from build123d import *

# Parameters (mm, degrees)
EXTRUDE_DEPTH                  = 30
EXTRUDE_ONTO_SKETCH_ROLL_ANGLE = 90


with BuildPart() as part:
    # Sketch as drawn → Extrude (new)
    with BuildSketch(Plane.XY):
        Polygon((-26.2, 22), (26.2, 22), (26.2, 0), (16.2, 0), (16.2, 12), (-16.2, 12), (-16.2, 0), (-26.2, 0), align=None)
    extrude(amount=-EXTRUDE_DEPTH)


with BuildPart() as part_1:
    # Extrude onto Sketch roll: moved
    add(part.part.rotate(Axis((0, 0, 0), (1, 0, 0)), EXTRUDE_ONTO_SKETCH_ROLL_ANGLE))


with BuildPart() as part_2:
    # Extrude onto Sketch placement: moved
    add(part_1.part)


solid = part_2.part
Geometry: final body of the model. Coordinates: model frame, mm. A direction names the side the tool comes from. Give positions to 0.01 mm unless a question says otherwise; leave off trailing zeros. Write each loop counter-clockwise with the first axis right and the second up, starting at its lowest first coordinate (ties: lowest second). Pieces come first, ordered by that corner, then holes.
(1) Access query for faces 4 (the flat face through (-21, 15, 0)), 5 (the flat face through (0, 15, 12)). Directions: +Z, -Z, +X, -X, +Y, -Y. A direction counts if a zero-diameter tool reaches every point of the face in a straight line with its end or side. Return the directions, or none.
(2) Ray query, line 1 (X direction, y = 28.5, z = 6.5); line 2 (Z direction, x = 15, y = 14). Return the intervals inside material, ascending.
(3) Cut plane A-A, the plane z = 9.5. Return loops of the section in (x, y), then the cut area to 3 significant figures.
(4) Cut plane C-C, the plane x = -7. Return loops of the section in (y, z), then the cut area to 3 significant figures.
(5) Mould query, pull axis X, two halves, no side actions, for faces 1 (the flat face through (26.2, 15, 11)), 2 (the flat face through (0, 15, 22)), 3 (the flat face through (16.2, 15, 6)). Classes: released by +X, released by -X, zero draft, split by the parting line, or undercut.
(6) First-contact query: P1, Ø15, axis at x = 5.5, y = 11.5, coming from the -Z side. Flat tip, straight axial feed; report the tip coordinate or a pass-through.
(7) Cut plane B-B, the plane y = 22. Return loops of the section in (x, z).
Values follow:
1. face 4: -Z, +X, -X, +Y, -Y
1. face 5: -Z, +Y, -Y
2. line 1: x = -26.2 to -16.2, 16.2 to 26.2
2. line 2: z = 12 to 22
3. outline: (-26.2, 0) - (-16.2, 0) - (-16.2, 30) - (-26.2, 30) - close; (16.2, 0) - (26.2, 0) - (26.2, 30) - (16.2, 30) - close
3. area: 600 mm2
4. outline: (0, 12) - (30, 12) - (30, 22) - (0, 22) - close
4. area: 300 mm2
5. face 1: released by +X
5. face 2: zero draft
5. face 3: undercut
6. P1: stops at z = 12
7. outline: (-26.2, 0) - (-16.2, 0) - (-16.2, 12) - (16.2, 12) - (16.2, 0) - (26.2, 0) - (26.2, 22) - (-26.2, 22) - close
